Build history of the part. All positions in model axes, mm. A direction names the side the tool comes from. Coordinates: 2 decimals unless noted, no trailing zeros. Loops run counter-clockwise (first coordinate to the right, second up) from the corner with the lowest first, then second, coordinate; pieces in that order, holes last.
Item 1: Flat gauge pins, fed straight in: pin 1 (10.5 mm diameter, centred on y = 0, z = 0, fed in from +X); pin 2 (6 mm diameter, centred on x = 5, z = -8, fed in from +Y); pin 3 (3.5 mm diameter, centred on x = 4, z = 8, fed in from -Y); pin 4 (7.5 mm diameter, centred on x = 26, z = 8, fed in from +Y). Where does each tip first touch, or does it go through?
Item 2: Mould opens along Y. For faces 4 (the face through (14.79, -11.09, -5.77)), 5 (the face through (8, 0, 3)), 6 (the face through (25.792, -3.012, 6.414)), 7 (the face through (15, 3, 1)) say: released by +Y, released by -Y, zero draft, split by the parting line, or undercut.
Item 3: Cut at A-A (y = 0). List the corners of the cut face in (x, z).
Item 4: Cut at D-D (z = 8). List the corners of the cut face in (x, y), and give its area (3 significant figures).
Item 5: 3-axis set-ups, long thin cutter, end or side, ignore diameter. For faces 1 (the face through (3.629, 7.227, 5.174)), 2 (the face through (22.605, -3.905, 0.867)), 3 (the face through (4.86, -3.01, 6.65)): which of +Z, -Z, +X, -X, +Y, -Y reach the whole face in a straight line?
Item 6: Cut at B-B (x = 26). List the corners of the cut face in (y, z), and give its area (3 significant figures).
Item 7: Cut at C-C (z = 0). List the corners of the cut face in (x, y).
Item 8: Drill centre lines: line 1 along X through (y, z) = (-3.5, 8); line 2 along X through (y, z) = (7.25, 8); line 3 along Z through (x, y) = (4, -1). Where is each one in solid material? Low to high.
from build123d import *

# Parameters (mm, degrees)
SKETCH_2_R                = 1.6
CUT_EXTRUDE_M3_DEPTH      = 13.5
CUT_EXTRUDE_M3_DEPTH_BACK = 13.5
SKETCH_3_R                = 2.85
CUT_EXTRUDE_993_DEPTH     = 8


with BuildPart() as part:
    # 草图1 → Revolve 643 (revolve)
    with BuildSketch(Plane(origin=(0, 0, 0), x_dir=(1, 0, 0), z_dir=(0, 1, 0))):
        Polygon((0, 12.5), (0, 3), (15, 3), (15, 4), (30, 4), (30, 12.5), align=None)
    revolve(axis=Axis((-118.9426696, 0, 0), (1, 0, 0)))

    # 草图2 → M3孔 (cut, two sides)
    with BuildSketch(Plane(origin=(0, 0, 0), x_dir=(1, 0, 0), z_dir=(0, 1, 0))) as cut_extrude_m3_sk:
        with Locations((4, -8)):
            Circle(SKETCH_2_R)
        with Locations((26, -8)):
            Circle(SKETCH_2_R)
    extrude(amount=CUT_EXTRUDE_M3_DEPTH, mode=Mode.SUBTRACT)
    extrude(cut_extrude_m3_sk.sketch, amount=-CUT_EXTRUDE_M3_DEPTH_BACK, mode=Mode.SUBTRACT)

    # 草图3 → Cut-Extrude 993 (cut)
    with BuildSketch(Plane(origin=(0, 12.499395806, 0), x_dir=(1, 0, 0), z_dir=(0, 1, 0))):
        with Locations((4, -8)):
            Circle(SKETCH_3_R)
        with Locations((26, -8)):
            Circle(SKETCH_3_R)
    extrude(amount=-CUT_EXTRUDE_993_DEPTH, mode=Mode.SUBTRACT)


solid = part.part
Filled sheet:
1. pin 1: stops at x = 30
1. pin 2: stops at y = 11.46
1. pin 3: stops at y = -10.83
1. pin 4: stops at y = 11.76
2. face 4: split by the parting line
2. face 5: undercut
2. face 6: zero draft
2. face 7: undercut
3. outline: (0, -12.5) - (30, -12.5) - (30, -4) - (15, -4) - (15, -3) - (0, -3) - close; (0, 3) - (15, 3) - (15, 4) - (30, 4) - (30, 12.5) - (0, 12.5) - close; hole circle Ø3.2 at (4, 8); hole circle Ø3.2 at (26, 8)
4. outline: (0, -9.6) - (2.4, -9.6) - (2.4, 4.5) - (1.15, 4.5) - (1.15, 9.6) - (0, 9.6) - close; (5.6, -9.6) - (24.4, -9.6) - (24.4, 4.5) - (23.15, 4.5) - (23.15, 9.6) - (6.85, 9.6) - (6.85, 4.5) - (5.6, 4.5) - close; (27.6, -9.6) - (30, -9.6) - (30, 9.6) - (28.85, 9.6) - (28.85, 4.5) - (27.6, 4.5) - close
4. area: 428 mm2
5. face 1: +Y
5. face 2: +X
5. face 3: +Y, -Y
6. outline: (-10.74, 6.4) arc R12.5 ccw (long way) to (11.39, 5.15) - (4.5, 5.15) - (4.5, 6.4) - close; (-8.01, 9.6) - (4.5, 9.6) - (4.5, 10.85) - (6.21, 10.85) arc R12.5 ccw to start; hole circle Ø8 at (0, 0)
6. area: 368 mm2
7. outline: (0, -12.5) - (30, -12.5) - (30, -4) - (15, -4) - (15, -3) - (0, -3) - close; (0, 3) - (15, 3) - (15, 4) - (30, 4) - (30, 12.5) - (0, 12.5) - close
8. line 1: x = 0 to 2.4, 5.6 to 24.4, 27.6 to 30
8. line 2: x = 0 to 1.15, 6.85 to 23.15, 28.85 to 30
8. line 3: z = -12.46 to -2.83, 2.83 to 6.4, 9.6 to 12.46
